Model file for the job. Use its own axes, mm. A direction names the side the tool comes from. Round coordinates to 2 decimals unless told otherwise and drop trailing zeros. Loops run counter-clockwise (first coordinate to the right, second up) from the corner with the lowest first, then second, coordinate; pieces in that order, holes last. Notation, with made-up numbers: M -39.5,64 L 14.5,64 A15 ccw 14.5,81 Z; hole C -22,55.25 d4. An arc over 180 degrees is marked long. Answer in a Markdown table with one row per item.
from build123d import *

# Parameters (mm, degrees)
BOSS_EXTRUDE1_DEPTH = 16
SKETCH1_3_W         = 10
SKETCH1_3_H         = 55.866863614
SKETCH1_3_R         = 2.85
BOSS_EXTRUDE2_DEPTH = 6
SKETCH1_4_R         = 2.85
SKETCH1_4_R_2       = 1.6
BOSS_EXTRUDE3_DEPTH = 2.5
CHAMFER3_SIZE       = 10.645574538
CHAMFER4_SIZE       = 9
CUT_EXTRUDE2_DEPTH  = 27.5
FILLET1_R           = 10


with BuildPart() as part:
    # Sketch1 → Boss-Extrude1 (new body)
    with BuildSketch(Plane(origin=(0, 0, 0), x_dir=(0, 1, 0), z_dir=(0, 0, 1))):
        with BuildLine():
            Line((-40.217333264, 33.746349509), (-37.536177713, 31.496592875))
            ThreePointArc((-37.536177713, 31.496592875), (-20.708294825, 44.409081565), (0, 49))
            Line((0, 49), (0, 52.5))
            Line((0, 52.5), (0, 59))
            ThreePointArc((0, 59), (-20.225540206, 55.42497202), (-38, 45.133136386))
            Line((-38, 45.133136386), (-48, 45.133136386))
            Line((-48, 45.133136386), (-48, 40.276782297))
            Line((-48, 40.276782297), (-40.217333264, 33.746349509))
        make_face()
    extrude(amount=BOSS_EXTRUDE1_DEPTH)

    # Sketch1<3> → Boss-Extrude2 (add)
    with BuildSketch(Plane(origin=(0, 0, 0), x_dir=(0, 1, 0), z_dir=(0, 0, 1))):
        with Locations((-43, 73.066568193)):
            Rectangle(SKETCH1_3_W, SKETCH1_3_H)
        with Locations(Location((-43, 96, 0), (0, 0, 270))):
            Circle(SKETCH1_3_R, mode=Mode.SUBTRACT)
        with Locations(Location((-43, 63, 0), (0, 0, 270))):
            Circle(SKETCH1_3_R, mode=Mode.SUBTRACT)
    extrude(amount=BOSS_EXTRUDE2_DEPTH)

    # Sketch1<4> → Boss-Extrude3 (add)
    # profile 1 of 2: a face of its own
    with BuildSketch(Plane(origin=(0, 0, 0), x_dir=(0, 1, 0), z_dir=(0, 0, 1))):
        with Locations(Location((-43, 96, 0), (0, 0, 270))):
            Circle(SKETCH1_4_R)
        with Locations(Location((-43, 96, 0), (0, 0, 270))):
            Circle(SKETCH1_4_R_2, mode=Mode.SUBTRACT)
    # profile 2 of 2: a face of its own
    with BuildSketch(Plane(origin=(0, 0, 0), x_dir=(0, 1, 0), z_dir=(0, 0, 1))):
        with Locations(Location((-43, 63, 0), (0, 0, 270))):
            Circle(SKETCH1_4_R)
        with Locations(Location((-43, 63, 0), (0, 0, 270))):
            Circle(SKETCH1_4_R_2, mode=Mode.SUBTRACT)
    extrude(amount=BOSS_EXTRUDE3_DEPTH)

    # Chamfer3
    # the kernel refuses this chamfer: 15, 10.645574538 mm, written as the material it adds along each edge
    with BuildSketch(Plane(origin=(-45.133136386, -38, 0), x_dir=(-0.520323475299402, 0.8539692506480269, 0), z_dir=(0, 0, 1))) as chamfer3_piece_1_section:
        with BuildLine():
            Line((17.934002299, 0), (CHAMFER3_SIZE * 0.520323475317, CHAMFER3_SIZE * 0.853969250677))
            Line((CHAMFER3_SIZE * 0.520323475317, CHAMFER3_SIZE * 0.853969250677), (0, 0))
            ThreePointArc((0, 0), (9.212497423, 0.684886528), (17.934002299, 0))
        make_face()
    chamfer3_piece_1 = extrude(amount=6, mode=Mode.PRIVATE)
    chamfer3_piece_1 = split(chamfer3_piece_1, bisect_by=Plane(origin=(-45.133136386, -38, 0), z_dir=(-1, 0, 0)), keep=Keep.TOP, mode=Mode.PRIVATE)
    add(chamfer3_piece_1)

    # Chamfer4
    chamfer4_edges = [part.edges().sort_by_distance(p)[0] for p in [
        (-45.133136386, -43, 6),
    ]]
    chamfer(chamfer4_edges, length=CHAMFER4_SIZE)

    # Sketch3 → Cut-Extrude2 (cut)
    with BuildSketch(Plane(origin=(-40.248296437, -18.768088856, 0), x_dir=(0, 0, -1), z_dir=(0.9063077870366554, 0.42261826174068795, 0))):
        with BuildLine():
            Line((-11.5, -15), (-11.5, -26.481070055))
            Line((-11.5, -26.481070055), (-21.940266499, -26.481070055))
            Line((-21.940266499, -26.481070055), (-21.940266499, 24.934477443))
            Line((-21.940266499, 24.934477443), (-11.5, 24.934477443))
            Line((-11.5, 24.934477443), (-11.5, 15))
            add(Edge.make_bspline(
                [(-11.5, -15), (-11.5, -10.5), (-14.436309762, -3.235504373), (-14.602449576, 2.674959083), (-11.5, 10.5), (-11.5, 15)],
                knots=[0, 0, 0, 0, 0.483457159, 0.583457159, 1, 1, 1, 1], degree=3))
        make_face()
    extrude(amount=-CUT_EXTRUDE2_DEPTH, mode=Mode.SUBTRACT)

    # Fillet1
    fillet1_edges = [part.edges().sort_by_distance(p)[0] for p in [
        (-55.778710924, -38, 3),
    ]]
    fillet(fillet1_edges, radius=FILLET1_R)


solid = part.part
1. Saw through at B-B (x = -96). Write the cut outline in (y, z).
Verdict:
| item | result |
|---|---|
| outline | M -48,0 L -44.6,0 L -44.6,2.5 L -45.85,2.5 L -45.85,6 L -48,6 Z; M -41.4,0 L -38,0 L -38,6 L -40.15,6 L -40.15,2.5 L -41.4,2.5 Z |
2. Saw through at A-A (z = 4). Write the cut outline in (x, y), and give its area (3 significant figures).
Verdict:
| item | result |
|---|---|
| outline | M -101,-48 L -40.28,-48 L -31.5,-37.54 A49 cw -49,0 L -59,0 A59 ccw -54.46,-22.68 L -54.99,-28.85 A10 cw -64.96,-38 L -101,-38 Z; hole C -96,-43 d5.7; hole C -63,-43 d5.7 |
| area | 1,110 mm² |
3. Pin check, flat tips, straight feed: pin 1 (4.5 mm diameter, centred on x = -63.5, y = -42, fed in from +Z); pin 2 (4.5 mm diameter, centred on x = -37, y = -40, fed in from +Z); pin 3 (1.5 mm diameter, centred on y = -30.5, z = 12, fed in from +X); pin 4 (3 mm diameter, centred on x = -63, y = -43, fed in from +Z). Stop position of each tip, or through.
Verdict:
| item | result |
|---|---|
| pin 1 | stops at z = 6 |
| pin 2 | stops at z = 11.5 |
| pin 3 | stops at x = -37.78 |
| pin 4 | passes through |
4. Saw through at C-C (y = -43). Write the cut outline in (x, z).
Verdict:
| item | result |
|---|---|
| outline | M -101,0 L -97.6,0 L -97.6,2.5 L -98.85,2.5 L -98.85,6 L -101,6 Z; M -94.4,0 L -64.6,0 L -64.6,2.5 L -65.85,2.5 L -65.85,6 L -93.15,6 L -93.15,2.5 L -94.4,2.5 Z; M -61.4,0 L -36.08,0 L -36.08,11.5 L -48.63,11.5 L -54.13,6 L -60.15,6 L -60.15,2.5 L -61.4,2.5 Z |
5. Tool access for faces 1 (the flat face through (-74, -42, 6)), 2 (the cylindrical face through (-57.365, -13.791, 7.149)), 3 (the flat face through (-54.726, -25.727, 2.958)), 4 (the flat face through (-63, -45, 2.5)): list every direction of +Z, -Z, +X, -X, +Y, -Y with a clear straight run to the whole face (end or side of a thin tool).
Verdict:
| item | result |
|---|---|
| face 1 | +Z, -X, -Y |
| face 2 | +Z, -X |
| face 3 | +Z, -Z, -X |
| face 4 | +Z |
6. Mould opens along Y. For faces 5 (the flat face through (-51.742, -38.63, 8.391)), 6 (the flat face through (-83, -38, 3)), 7 (the flat face through (-96, -45, 2.5)), 8 (the cylindrical face through (-62.26, -44.42, 1.23)) say: +Y half, -Y half, draft (parallel to the pull), parting line (faces both ways), or undercut.
Verdict:
| item | result |
|---|---|
| face 5 | draft |
| face 6 | +Y half |
| face 7 | undercut |
| face 8 | undercut |
7. Saw through at D-D (z = 8). Write the cut outline in (x, y).
Verdict:
| item | result |
|---|---|
| outline | M -59,0 A59 ccw -52.13,-27.62 L -52.13,-48 L -40.28,-48 L -31.5,-37.54 A49 cw -49,0 Z |
8. Wall check: probe 1 along Z at (x, y) = (-77, -43); probe 2 along Y at (x, z) = (-95, 4); probe 3 along Y at (x, z) = (-64.5, 4.75). Give the ranges that are in metal, low to high.
Verdict:
| item | result |
|---|---|
| probe 1 | z = 0 to 6 |
| probe 2 | y = -48 to -45.67, -40.33 to -38 |
| probe 3 | y = -48 to -45.42, -40.58 to -37.99 |
